```python
from build123d import *

# Parameters (mm, degrees)
PAD_DEPTH    = 15
SKETCH001_R  = 3.5
PAD001_DEPTH = 15


with BuildPart() as part:
    # Sketch → Pad (new body)
    with BuildSketch(Plane.XY):
        Polygon((0, 0), (-5, 0), (-5, 15), (-57.980821, 5.658052), (-60.238248, 18.460553), (-56.299017, 19.155145), (-54.562535, 9.307068), (13.3892, 21.288792), (13.3892, 18.288792), (0, 15.927915), align=None)
    extrude(amount=PAD_DEPTH)

    # Sketch001 → Pad001 (new body)
    with BuildSketch(Plane.YZ):
        with Locations((18.460553, 15)):
            Circle(SKETCH001_R)
    extrude(amount=-PAD001_DEPTH)


solid = part.part
```
Part model, mm, in its own coordinate system. A direction names the side the tool comes from. Give positions to 0.01 mm unless a question says otherwise; leave off trailing zeros. Order: outer loops, then holes, each group sorted by start corner. A loop starts at its lowest first (then second) coordinate and runs counter-clockwise, first axis right, second up. Notation, with made-up numbers: M -10.75,27.5 L -0.75,27.5 A11 cw -0.75,37.5 Z; hole C 56.25,31.5 d9. An arc over 180 degrees is marked long. Use a Markdown table: item, result. Add a question column.
(1) Probe line 1 along Z through (x, y) = (-23.5, 14.25); line 2 along X through (y, z) = (3.25, 1.25); line 3 along X through (y, z) = (19.75, 17.5). List the from-to ranges inside material, lowest first. Write a range as [from, to].
(2) Saw through at A-A, the plane y = 6.5. Give the cut face in (x, z), and give its area (3 significant figures).
(3) Mould opens along X. For faces 1 (the face through (-23, 13, 0)), 2 (the face through (-31.12, 10.394, 7.395)), 3 (the face through (-55.443, 14.3, 7.395)), 4 (the face through (13.389, 20, 7)) say: +X half, -X half, draft (parallel to the pull), parting line (faces both ways), or undercut.
(4) 3-axis set-ups, long thin cutter, end or side, ignore diameter. For faces 5 (the face through (-5, 7, 7)), 6 (the face through (6.788, 17.125, 7.395)), 7 (the face through (-2, 8, 15)), 8 (the face through (7, 19, 15)): which of +Z, -Z, +X, -X, +Y, -Y reach the whole face in a straight line?
(5) Saw through at B-B, the plane z = 8. Give the cut face in (x, y), and give its area (3 significant figures).
(6) Drop flat-ended pins along their axis: P1, Ø1.5, axis at x = -2, y = 7, coming from the +Z side; P2, Ø1, axis at y = 8.5, z = 9.5, coming from the +X side; P3, Ø7.5, axis at y = 5, z = 9.5, coming from the -X side. Give the stop position or say it passes through.
(7) Saw through at D-D, the plane x = 2. Give the cut face in (y, z).
(8) Saw through at C-C, the plane y = 13.25. Give the cut face in (x, z).
Answer key:
| question | item | result |
|---|---|---|
| 1 | line 1 | [0, 15] |
| 1 | line 2 | [-5, 0] |
| 1 | line 3 | [-15, 0] |
| 2 | outline | M -58.13,0 L -53.21,0 L -53.21,15 L -58.13,15 Z; M -5,0 L 0,0 L 0,15 L -5,15 Z |
| 2 | area | 149 mm^2 |
| 3 | face 1 | draft |
| 3 | face 2 | undercut |
| 3 | face 3 | undercut |
| 3 | face 4 | +X half |
| 4 | face 5 | +Z, -Z, -Y |
| 4 | face 6 | +Z, -Z, +X, -Y |
| 4 | face 7 | +Z, +X, -X, -Y |
| 4 | face 8 | +Z, +X, +Y, -Y |
| 5 | outline | M -60.24,18.46 L -57.98,5.66 L -5,15 L -5,0 L 0,0 L 0,15.93 L 13.39,18.29 L 13.39,21.29 L -54.56,9.31 L -56.3,19.16 Z |
| 5 | area | 335 mm^2 |
| 6 | P1 | z = 15 |
| 6 | P2 | x = 0 |
| 6 | P3 | x = -58.53 |
| 7 | outline | M 16.28,0 L 19.28,0 L 19.28,15 L 16.28,15 Z |
| 8 | outline | M -59.32,0 L -55.26,0 L -55.26,15 L -59.32,15 Z; M -32.2,0 L -14.92,0 L -14.92,15 L -32.2,15 Z; M -5,0 L 0,0 L 0,15 L -5,15 Z |
